from build123d import *

# Parameters (mm, degrees)
BOSS_EXTRUDE1_DEPTH = 11.5
BOSS_EXTRUDE2_DEPTH = 26.3
BOSS_EXTRUDE3_DEPTH = 10
SKETCH4_W           = 10
SKETCH4_H           = 0.6
SKETCH5_W           = 10
SKETCH5_H           = 0.6
SKETCH6_W           = 10
SKETCH6_H           = 0.6
SKETCH7_W           = 10
SKETCH7_H           = 0.6
HOLE1_D             = 2.459
HOLE1_DEPTH         = 5
HOLE2_D             = 2.459
HOLE2_DEPTH         = 5
HOLE3_D             = 2.459
HOLE3_DEPTH         = 5
HOLE4_D             = 2.459
HOLE4_DEPTH         = 5


with BuildPart() as part:
    # Sketch1 → Boss-Extrude1 (new body)
    with BuildSketch(Plane(origin=(0, 0, 0), x_dir=(-1, 0, 0), z_dir=(0, 0, -1))):
        Polygon((-15.828427125, 21), (-21, 15.828427125), (-21, -15.828427125), (-15.828427125, -21), (15.828427125, -21), (21, -15.828427125), (21, 15.828427125), (15.828427125, 21), align=None)
    extrude(amount=-BOSS_EXTRUDE1_DEPTH)

    # Sketch2 → Boss-Extrude2 (add)
    with BuildSketch(Plane.XY.offset(11.5)):
        Polygon((13, -21), (-13, -21), (-21, -13), (-21, 13), (-13, 21), (13, 21), (21, 13), (21, -13), align=None)
    extrude(amount=BOSS_EXTRUDE2_DEPTH)

    # Sketch3 → Boss-Extrude3 (add)
    with BuildSketch(Plane.XY.offset(37.8)):
        Polygon((15.828427125, 21), (21, 15.828427125), (21, -15.828427125), (15.828427125, -21), (-15.828427125, -21), (-21, -15.828427125), (-21, 15.828427125), (-15.828427125, 21), align=None)
    extrude(amount=BOSS_EXTRUDE3_DEPTH)

    # Sketch4 → Revolve1 (revolve)
    with BuildSketch(Plane.XY.offset(3.65)):
        with Locations((-26, 0.95)):
            Rectangle(SKETCH4_W, SKETCH4_H)
    revolve(axis=Axis((-31, 0.65, 3.65), (1, 0, 0)))

    # Sketch5 → Revolve2 (revolve)
    with BuildSketch(Plane.XY.offset(3.65)):
        with Locations((-26, -0.35)):
            Rectangle(SKETCH5_W, SKETCH5_H)
    revolve(axis=Axis((-31, -0.65, 3.65), (1, 0, 0)))

    # Sketch6 → Revolve3 (revolve)
    with BuildSketch(Plane.XY.offset(4.95)):
        with Locations((-26, -0.35)):
            Rectangle(SKETCH6_W, SKETCH6_H)
    revolve(axis=Axis((-31, -0.65, 4.95), (1, 0, 0)))

    # Sketch7 → Revolve4 (revolve)
    with BuildSketch(Plane.XY.offset(4.95)):
        with Locations((-26, 0.95)):
            Rectangle(SKETCH7_W, SKETCH7_H)
    revolve(axis=Axis((-31, 0.65, 4.95), (1, 0, 0)))

    # Sketch8 → Revolve5 (revolve)
    with BuildSketch(Plane.XZ):
        Polygon((2.5, 71.8), (0, 71.8), (0, 47.8), (11, 47.8), (11, 49.8), (2.5, 49.8), align=None)
    revolve(axis=Axis((0, 0, 71.8), (0, 0, -1)))

    # Hole1
    with Locations(Plane.XY.offset(47.8)):
        with Locations((-15.5, 15.5)):
            Hole(HOLE1_D / 2, depth=HOLE1_DEPTH)

    # Hole2
    with Locations(Plane.XY.offset(47.8)):
        with Locations((-15.5, -15.5)):
            Hole(HOLE2_D / 2, depth=HOLE2_DEPTH)

    # Hole3
    with Locations(Plane.XY.offset(47.8)):
        with Locations((15.5, 15.5)):
            Hole(HOLE3_D / 2, depth=HOLE3_DEPTH)

    # Hole4
    with Locations(Plane.XY.offset(47.8)):
        with Locations((15.5, -15.5)):
            Hole(HOLE4_D / 2, depth=HOLE4_DEPTH)


solid = part.part
Check sheet for the modelled part. Datum: model origin and axes. Units: mm. A direction names the side the tool comes from. Round coordinates to 2 decimals unless told otherwise and drop trailing zeros. Order: outer loops, then holes, each group sorted by start corner. A loop starts at its lowest first (then second) coordinate and runs counter-clockwise, first axis right, second up.
Q1. Set-up check for faces 4 (the face through (16, -15, 42.8)), 5 (the face through (18, 18, 37.8)), 6 (the face through (18, -18, 11.5)): record each of +Z, -Z, +X, -X, +Y, -Y from which the full face is reachable in a straight line by a thin tool's end or side.
Filled sheet:
face 4: +Z
face 5: +X, +Y
face 6: +X, -Y
Q2. Cross-section at B-B, the plane x = 0. Enter the section's corners in (y, z).
Filled sheet:
outline: (-21, 0) - (21, 0) - (21, 47.8) - (11, 47.8) - (11, 49.8) - (2.5, 49.8) - (2.5, 71.8) - (-2.5, 71.8) - (-2.5, 49.8) - (-11, 49.8) - (-11, 47.8) - (-21, 47.8) - close
Q3. Cross-section at A-A, the plane z = 44.5. Enter the section's corners in (x, y).
Filled sheet:
outline: (-21, -15.83) - (-15.83, -21) - (15.83, -21) - (21, -15.83) - (21, 15.83) - (15.83, 21) - (-15.83, 21) - (-21, 15.83) - close; hole circle Ø2.46 at (-15.5, -15.5); hole circle Ø2.46 at (-15.5, 15.5); hole circle Ø2.46 at (15.5, -15.5); hole circle Ø2.46 at (15.5, 15.5)
Q4. Cross-section at C-C, the plane z = 13. Enter the section's corners in (x, y), plus the area to 3 significant figures.
Filled sheet:
outline: (-21, -13) - (-13, -21) - (13, -21) - (21, -13) - (21, 13) - (13, 21) - (-13, 21) - (-21, 13) - close
area: 1,640 mm2
Q5. Depth check by flat-ended pin: P1, Ø5, axis at y = -10.5, z = 37.5, coming from the -X side; P2, Ø8, axis at x = -23, z = 30.5, coming from the +Y side; P3, Ø0.7, axis at x = 15, y = -15.5, coming from the +Z side. Enter the tip coordinate at first touch or a pass-through.
Filled sheet:
P1: stops at x = -21
P2: stops at y = 15
P3: stops at z = 42.8
Q6. Scan lines: L1, parallel to Y at x = 15.5, z = 46.05; L2, parallel to X at y = -15, z = 44; L3, parallel to Z at x = -17, y = 19. Record each from-to range of solid material in increasing order.
Filled sheet:
L1: y = -21 to -16.73, -14.27 to 14.27, 16.73 to 21
L2: x = -21 to -16.62, -14.38 to 14.38, 16.62 to 21
L3: z = 0 to 11.5, 37.8 to 47.8
Q7. Cross-section at D-D, the plane y = -4. Enter the section's corners in (x, z), plus the area to 3 significant figures.
Filled sheet:
outline: (-21, 0) - (21, 0) - (21, 47.8) - (10.25, 47.8) - (10.25, 49.8) - (-10.25, 49.8) - (-10.25, 47.8) - (-21, 47.8) - close
area: 2,050 mm2
Q8. Draft check along Z on faces 1 (the face through (-18, -18, 11.5)), 2 (the face through (0, 0, 0)), 3 (the face through (-18.38, -18.45, 42.73)). Enter one of: pulls with the +Z half, pulls with the -Z half, needs draft (parallel to the pull), parting line crosses it, or undercut.
Filled sheet:
face 1: undercut
face 2: pulls with the -Z half
face 3: needs draft
